Source: CAD feature listing. Evaluate the final solid. Frame: model axes, mm. Round coordinates to 2 decimals unless told otherwise and drop trailing zeros. Loops run counter-clockwise (first coordinate to the right, second up) from the corner with the lowest first, then second, coordinate; pieces in that order, holes last. Notation, with made-up numbers: (25.5, 75.5) - (55.5, 75.5) arc R10 cw to (55.5, 91.5) - close; hole circle Ø1 at (-26.75, 72.25). An arc over 180 degrees is marked (long way). One line per question, with ' | ' between items.
Autodesk Fusion 360 part; units mm, degrees
sketch "Sketch1" plane through (0, 0, 0) normal (0, 0, 1) x (1, 0, 0)
  circle A0 centre (0, 0) radius 3.175
  dimension "d1" = 6.35
extrude "Extrude1" add sketch "Sketch1" along normal blind 8
sketch "Sketch2" plane through (0, 0, 8) normal (0, 0, 1) x (-1, 0, 0)
  circle A0 centre (0, 0) radius 3.175
  circle A1 centre (0, 0) radius 2
hole "Hole1" at (0, 0, 8) direction (0, 0, -1) diameter 4.234 depth 8 tip angle 180
sketch "Sketch4" plane through (0, 0, 0) normal (1, 0, 0) x (0, 1, 0)
  line L0 (3.175, 8) -> (-3.175, 8)
sketch "Sketch5" plane through (0, 0, 0) normal (0, 0, -1) x (1, 0, 0)
  circle A0 centre (0, 0) radius 2.117
  circle A1 centre (0, 0) radius 3.175
  circle A2 centre (0, 0) radius 3.5
  circle A3 centre (0, 0) radius 2.117
  circle A4 centre (0, 0) radius 1.1
  dimension "d17" = 7
  dimension "d18" = 4.234
  dimension "d19" = 2.2
extrude "Extrude3" add sketch "Sketch5" against normal blind 1.2 contours A0 A3
sketch "Sketch3" plane through (0, 0, 0) normal (0, 1, 0) x (1, 0, 0)
  line L0 (-0.5, -0.1) -> (0.5, -0.1)
  line L1 (0.5, -0.1) -> (0.5, -1.1)
  line L2 (0.5, -1.1) -> (-0.5, -1.1)
  line L3 (-0.5, -1.1) -> (-0.5, -0.1)
  line L4 (0, -1.75) -> (0, -22.5)
  line L5 (1.75, 0) -> (22.5, 0)
  circle A0 centre (0, -0.5996) radius 0.4064
  line L6 (0, -0.5996) -> (0, -1.1) construction
  line L7 (-0.35, -0.8061) -> (-0.35, -0.393)
  line L8 (0.35, -0.8061) -> (0.35, -0.393)
  dimension "d9" = 1
  dimension "d10" = 1
  dimension "d15" = 0.1
  dimension "d16" = 0.8128
  dimension "d24" = 0.4996
  dimension "d25" = 0.35
extrude "Extrude2" cut sketch "Sketch3" along normal mid plane 9 contours A0 L7 L8
fillet "Fillet2" [suppressed]
1. Contact query for flat-ended pins moving along their axis: P1, Ø2, axis at x = 0, y = 0, coming from the +Z side; P2, Ø0.5, axis at y = 2, z = 0.5, coming from the -X side; P3, Ø1.5, axis at x = 2.5, z = 1.5, coming from the +Y side. Output: stop coordinate, or through.
Worked out:
P1: passes through | P2: stops at x = -2.65 | P3: stops at y = 2.65
2. Material intervals for probe 1 along Z at (x, y) = (0, 3); probe 2 along Z at (x, y) = (0, 2); probe 3 along Z at (x, y) = (0.75, 1.25), sorted ascending.
Worked out:
probe 1: z = 0 to 0.19, 1.01 to 8 | probe 2: z = 0 to 0.19, 1.01 to 1.2 | probe 3: z = 0 to 1.2
3. Section query C-C, the plane y = -2.5. Return loops of the section in (x, z).
Worked out:
outline: (-1.96, 0) - (1.96, 0) - (1.96, 8) - (-1.96, 8) - close; hole (-0.35, 0.39) arc R0.41 ccw to (0.35, 0.39) - (0.35, 0.81) arc R0.41 ccw to (-0.35, 0.81) - close
4. Section query A-A, the plane y = 0. Return loops of the section in (x, z) (3 decimals).
Worked out:
outline: (-3.175, 0) - (-1.1, 0) - (-1.1, 1.2) - (-2.117, 1.2) - (-2.117, 8) - (-3.175, 8) - close; (1.1, 0) - (3.175, 0) - (3.175, 8) - (2.117, 8) - (2.117, 1.2) - (1.1, 1.2) - close
5. Section query B-B, the plane x = 0. Return loops of the section in (y, z) (3 decimals), plus the area to 3 significant figures.
Worked out:
outline: (-3.175, 0) - (-1.1, 0) - (-1.1, 0.193) - (-3.175, 0.193) - close; (-3.175, 1.006) - (-1.1, 1.006) - (-1.1, 1.2) - (-2.117, 1.2) - (-2.117, 8) - (-3.175, 8) - close; (1.1, 0) - (3.175, 0) - (3.175, 0.193) - (1.1, 0.193) - close; (1.1, 1.006) - (3.175, 1.006) - (3.175, 8) - (2.117, 8) - (2.117, 1.2) - (1.1, 1.2) - close | area: 16.0 mm2
6. Mould query, pull axis X, two halves, no side actions, for faces 1 (the cylindrical face through (-0.69, 3.1, 3.94)), 2 (the cylindrical face through (1.05, -0.33, 0.59)), 3 (the flat face through (1.4, 0, 0)). Classes: released by +X, released by -X, zero draft, split by the parting line, or undercut.
Worked out:
face 1: split by the parting line | face 2: undercut | face 3: zero draft
7. Section query D-D, the plane z = 4.5. Return loops of the section in (x, y) (3 decimals), plus the area to 3 significant figures.
Worked out:
outline: circle Ø6.35 at (0, 0); hole circle Ø4.234 at (0, 0) | area: 17.6 mm2
